Geometry check sheet. Reference: the model listing, model coordinates, mm. Give positions to 0.01 mm unless a question says otherwise; leave off trailing zeros. Order: outer loops, then holes, each group sorted by start corner. A loop starts at its lowest first (then second) coordinate and runs counter-clockwise, first axis right, second up. Notation, with made-up numbers: M 33.5,-8.75 L 91.5,-8.75 A17 cw 91.5,-2.75 Z; hole C 1.5,32.25 d3. An arc over 180 degrees is marked long. Answer as CSV lines item,"result". Start each with the question number.
Q1. Section check A-A, the plane y = -112.5. Record the boundary of the cut face in (x, z).
Q2. Section check C-C, the plane z = -1.15. Record the boundary of the cut face in (x, y), then the cut area to 3 significant figures.
Q3. Thickness scan on line 1 (Y direction, x = 22.5, z = -1.5); line 2 (X direction, y = -22, z = -1.6); line 3 (X direction, y = -67.5, z = -1.25). Record the ranges inside material, lowest first.
Q4. Mould release check, pull along X, two halves, no side actions. Record for faces 1 (the flat face through (113, -46, -1)), 2 (the flat face through (53, -68, 0)), 3 (the cylindrical face through (65.081, -116.294, -0.986)): +X half, -X half, draft (parallel to the pull), parting line (faces both ways), or undercut.
Q5. Section check B-B, the plane x = 112.5. Record the boundary of the cut face in (y, z), then the cut area to 3 significant figures.
Q6. Go/stop test with a flat-tipped pin: pin 1 (4 mm diameter, centred on x = 115, y = -79.5, fed in from +Z). Record where the tip stops, or that it passes through.
Q7. Section check D-D, the plane y = -22.5. Record the boundary of the cut face in (x, z).
```python
from build123d import *

# Parameters (mm, degrees)
EXTRUDE_1_DEPTH   = 2
HOLE_WIZARD_M81_D = 9
CHAMFER_1_SIZE    = 2


with BuildPart() as part:
    # Эскиз1 → Бобышка-Вытянуть1 (new body)
    with BuildSketch(Plane(origin=(0, 0, 0), x_dir=(1, 0, 0), z_dir=(0, 0, -1))):
        Polygon((0, 0), (0, 135), (135, 135), (135, 90), (90, 0), align=None)
    extrude(amount=EXTRUDE_1_DEPTH)

    # Отверстие с зазором M81 (through all)
    with Locations(Plane(origin=(0, 0, -2), x_dir=(1, 0, 0), z_dir=(0, 0, -1))):
        with Locations((67.5, 112.5), (22.5, 112.5), (22.5, 67.5), (22.5, 22.5), (112.5, 112.5), (67.5, 67.5), (67.5, 22.5)):
            Hole(HOLE_WIZARD_M81_D / 2)

    # Фаска1
    chamfer_1_edges = [part.edges().sort_by_distance(p)[0] for p in [
        (0, 0, -1),
        (0, -135, -1),
        (135, -135, -1),
    ]]
    chamfer(chamfer_1_edges, length=CHAMFER_1_SIZE)


solid = part.part
```
Answer block:
1,outline,"M 0,-2 L 18,-2 L 18,0 L 0,0 Z; M 27,-2 L 63,-2 L 63,0 L 27,0 Z; M 72,-2 L 108,-2 L 108,0 L 72,0 Z; M 117,-2 L 135,-2 L 135,0 L 117,0 Z"
2,outline,"M 0,-133 L 2,-135 L 133,-135 L 135,-133 L 135,-90 L 90,0 L 2,0 L 0,-2 Z; hole C 22.5,-112.5 d9; hole C 22.5,-67.5 d9; hole C 22.5,-22.5 d9; hole C 67.5,-112.5 d9; hole C 67.5,-67.5 d9; hole C 67.5,-22.5 d9; hole C 112.5,-112.5 d9"
2,area,"15,700 mm2"
3,line 1,"y = -135 to -117, -108 to -72, -63 to -27, -18 to 0"
3,line 2,"x = 0 to 18.03, 26.97 to 63.03, 71.97 to 101"
3,line 3,"x = 0 to 18, 27 to 63, 72 to 123.75"
4,face 1,"+X half"
4,face 2,"draft"
4,face 3,"undercut"
5,outline,"M -135,-2 L -117,-2 L -117,0 L -135,0 Z; M -108,-2 L -45,-2 L -45,0 L -108,0 Z"
5,area,"162 mm2"
6,pin 1,"stops at z = 0"
7,outline,"M 0,-2 L 18,-2 L 18,0 L 0,0 Z; M 27,-2 L 63,-2 L 63,0 L 27,0 Z; M 72,-2 L 101.25,-2 L 101.25,0 L 72,0 Z"
